Source: CAD feature listing. Evaluate the final solid. Frame: model axes, mm. A direction names the side the tool comes from. Coordinates: 2 decimals unless noted, no trailing zeros. Order: outer loops, then holes, each group sorted by start corner. A loop starts at its lowest first (then second) coordinate and runs counter-clockwise, first axis right, second up.
Autodesk Inventor part; units mm, degrees
ref_plane "YZ Plane" through (0, 0, 0) normal (1, 0, 0) x (0, 1, 0)
ref_plane "XZ Plane" through (0, 0, 0) normal (0, 1, 0) x (-1, 0, 0)
ref_plane "XY Plane" through (0, 0, 0) normal (0, 0, 1) x (1, 0, 0)
sketch "Skizze1" plane through (0, 0, 0) normal (0, 0, 1) x (1, 0, 0)
  line L0 (-13.335, 10.16) -> (13.335, 10.16)
  line L1 (13.335, 10.16) -> (13.335, -10.16)
  line L2 (13.335, -10.16) -> (-13.335, -10.16)
  line L3 (-13.335, -10.16) -> (-13.335, 10.16)
  line L4 (-13.335, 10.16) -> (13.335, -10.16) construction
  line L5 (13.335, 10.16) -> (-13.335, -10.16) construction
  point P0 (0, 0)
  dimension "d0" = 26.67
  dimension "d1" = 20.32
extrude "Extrusion1" add sketch "Skizze1" along normal blind 2
fillet "Rundung1" radius 2 4 edges at (-13.335, -10.16, 1) (13.335, -10.16, 1) (13.335, 10.16, 1) (-13.335, 10.16, 1)
sketch "Skizze2" plane through (0, 0, 0) normal (0, 0, -1) x (-1, 0, 0)
  line L0 (-10.795, -7.62) -> (10.795, -7.62) construction
  line L1 (10.795, -7.62) -> (10.795, 7.62) construction
  line L2 (10.795, 7.62) -> (-10.795, 7.62) construction
  line L3 (-10.795, 7.62) -> (-10.795, -7.62) construction
  line L4 (-10.795, -7.62) -> (10.795, 7.62) construction
  line L5 (10.795, -7.62) -> (-10.795, 7.62) construction
  line L6 (-6.35, -8.89) -> (6.35, -8.89) construction
  line L7 (6.35, -8.89) -> (6.35, 8.89) construction
  line L8 (6.35, 8.89) -> (-6.35, 8.89) construction
  line L9 (-6.35, 8.89) -> (-6.35, -8.89) construction
  line L10 (-6.35, -8.89) -> (6.35, 8.89) construction
  line L11 (6.35, -8.89) -> (-6.35, 8.89) construction
  circle A0 centre (6.35, 8.89) radius 0.5
  circle A1 centre (3.81, 8.89) radius 0.5
  line L12 (3.81, 8.89) -> (-8.89, 8.89) construction
  circle A2 centre (1.27, 8.89) radius 0.5
  line L13 (1.27, 8.89) -> (-11.43, 8.89) construction
  circle A3 centre (-1.27, 8.89) radius 0.5
  line L14 (-1.27, 8.89) -> (-13.97, 8.89) construction
  circle A4 centre (-3.81, 8.89) radius 0.5
  line L15 (-3.81, 8.89) -> (-16.51, 8.89) construction
  circle A5 centre (-6.35, 8.89) radius 0.5
  line L16 (-6.35, 8.89) -> (-19.05, 8.89) construction
  circle A6 centre (3.81, -8.89) radius 0.5
  circle A7 centre (1.27, -8.89) radius 0.5
  line L17 (-8.89, -8.89) -> (3.81, -8.89) construction
  circle A8 centre (-1.27, -8.89) radius 0.5
  line L18 (-11.43, -8.89) -> (1.27, -8.89) construction
  circle A9 centre (-3.81, -8.89) radius 0.5
  line L19 (-13.97, -8.89) -> (-1.27, -8.89) construction
  circle A10 centre (10.795, -7.62) radius 1.05
  circle A11 centre (-10.795, -7.62) radius 1.05
  circle A12 centre (-10.795, 7.62) radius 1.05
  circle A13 centre (10.795, 7.62) radius 1.05
  point P0 (0, 0)
  dimension "d5" = 21.59
  dimension "d6" = 15.24
  dimension "d7" = 17.78
  dimension "d8" = 12.7
  dimension "d9" = 1
  dimension "d14" = 2.54
  dimension "d19" = 1
  dimension "d22" = 2.54
  dimension "d27" = 2.1
  dimension "d28" = 2.1
  dimension "d29" = 2.1
  dimension "d30" = 2.1
extrude "Extrusion2" cut sketch "Skizze2" against normal through all
sketch "Skizze3" plane through (0, 0, 2) normal (0, 0, 1) x (1, 0, 0)
  line L0 (-3, 2) -> (3, 2)
  line L1 (3, 2) -> (3, -2)
  line L2 (3, -2) -> (-3, -2)
  line L3 (-3, -2) -> (-3, 2)
  line L4 (-3, 2) -> (3, -2) construction
  line L5 (3, 2) -> (-3, -2) construction
  point P0 (0, 0)
  dimension "d33" = 6
  dimension "d34" = 4
extrude "Extrusion3" add sketch "Skizze3" along normal blind 1.5
properties part number "BNO055" material "Kupfer, Guss"
1. Contact query for flat-ended pins moving along their axis: P1, Ø1.3, axis at x = -10.795, y = 7.62, coming from the -Z side; P2, Ø1.5, axis at x = -2, y = -6, coming from the +Z side. Output: stop coordinate, or through.
2. Access query for faces 1 (the cylindrical face through (-9.746, 7.666, 0.986)), 2 (the flat face through (3, 0, 3)). Directions: +Z, -Z, +X, -X, +Y, -Y. A direction counts if a zero-diameter tool reaches every point of the face in a straight line with its end or side. Return the directions, or none.
3. Draft query along Y for faces 3 (the flat face through (0, -10.16, 1)), 4 (the cylindrical face through (9.825, 7.218, 0.986)), 5 (the flat face through (0, 0, 0)). Return one class per face: +Y half, -Y half, draft (parallel to the pull), parting line (faces both ways), or undercut.
4. Section query D-D, the plane z = 0.9. Count the separate pieces of the cut face and the enclosed holes in it, plus the area to 3 significant figures.
5. Section query C-C, the plane y = -7.62. Output: boundary loops of the cut face in (x, z) (3 decimals), plus the area to 3 significant figures.
6. Material intervals for line 1 along Y through (x, z) = (-1.27, 1.3); line 2 along Y through (x, z) = (10.75, 1.5); line 3 along X through (y, z) = (-9, 0.3), sorted ascending.
7. Section query A-A, the plane x = 1.27. Output: boundary loops of the cut face in (y, z).
8. Section query B-B, the plane x = -6.35. Output: boundary loops of the cut face in (y, z), plus the area to 3 significant figures.
Answer key:
1. P1: passes through
1. P2: stops at z = 2
2. face 1: +Z, -Z
2. face 2: +Z, +X, +Y, -Y
3. face 3: -Y half
3. face 4: undercut
3. face 5: draft
4. separate pieces: 1
4. enclosed holes: 14
4. area: 517 mm2
5. outline: (-13.335, 0) - (-11.845, 0) - (-11.845, 2) - (-13.335, 2) - close; (-9.745, 0) - (9.745, 0) - (9.745, 2) - (-9.745, 2) - close; (11.845, 0) - (13.335, 0) - (13.335, 2) - (11.845, 2) - close
5. area: 44.9 mm2
6. line 1: y = -10.16 to -9.39, -8.39 to 8.39, 9.39 to 10.16
6. line 2: y = -10.16 to -8.67, -6.57 to 6.57, 8.67 to 10.16
6. line 3: x = -13.15 to -4.3, -3.32 to -1.76, -0.78 to 0.78, 1.76 to 3.32, 4.3 to 13.15
7. outline: (-10.16, 0) - (-9.39, 0) - (-9.39, 2) - (-10.16, 2) - close; (-8.39, 0) - (8.39, 0) - (8.39, 2) - (2, 2) - (2, 3.5) - (-2, 3.5) - (-2, 2) - (-8.39, 2) - close; (9.39, 0) - (10.16, 0) - (10.16, 2) - (9.39, 2) - close
8. outline: (-10.16, 0) - (8.39, 0) - (8.39, 2) - (-10.16, 2) - close; (9.39, 0) - (10.16, 0) - (10.16, 2) - (9.39, 2) - close
8. area: 38.6 mm2
